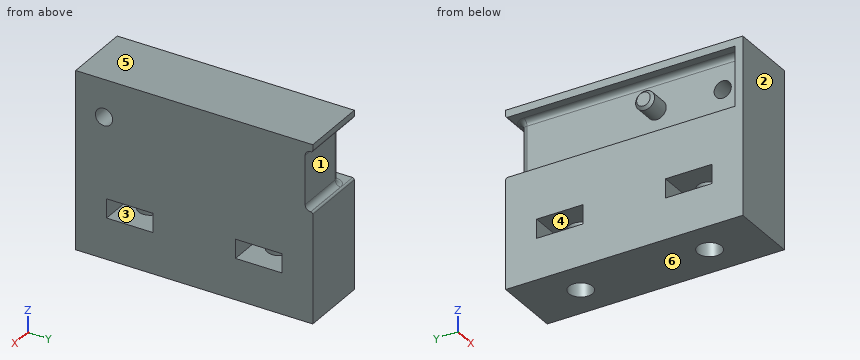
from build123d import *

# Parameters (mm, degrees)
F0_W      = 41
F0_H      = 11
F0_R      = 1.5875
F0_R_2    = 1.75
F1_DEPTH  = 10
F2_DEPTH  = 12.5
F3_R      = 1
F4_DEPTH  = 14
F5_SIZE   = 0.5
F6_DEPTH  = 19
F7_R      = 2.2
F8_DEPTH  = 20
F9_W      = 8.55
F9_H      = 3.5222247243
F10_DEPTH = 22.3


with BuildPart() as f1:
    # F0 (on Right) → F1 (new body)
    with BuildSketch(Plane.YZ):
        Rectangle(F0_W, F0_H)
        with Locations((-16.6625, 0)):
            Circle(F0_R, mode=Mode.SUBTRACT)
        with Locations((-4.475, 0)):
            Circle(F0_R_2, mode=Mode.SUBTRACT)
    extrude(amount=-F1_DEPTH)

    # F0 (on Right) → F2 (join)
    with BuildSketch(Plane.YZ):
        with BuildLine():
            Line((-20.5, 5.5), (20.5, 5.5))
            Line((20.5, 5.5), (21.5708505204, 5.5))
            ThreePointArc((21.5708505204, 5.5), (21.8035943853, 5.5964056654), (21.9000000507, 5.8291495303))
            Line((21.9000000507, 5.8291495303), (21.9000000507, 6.9000000507))
            Line((21.9000000507, 6.9000000507), (-21.9000000507, 6.9000000507))
            Line((-21.9000000507, 6.9000000507), (-21.9000000507, -6.9000000507))
            Line((-21.9000000507, -6.9000000507), (21.9000000507, -6.9000000507))
            Line((21.9000000507, -6.9000000507), (21.9000000507, -5.8291495303))
            ThreePointArc((21.9000000507, -5.8291495303), (21.8035943853, -5.5964056654), (21.5708505204, -5.5))
            Line((21.5708505204, -5.5), (20.5, -5.5))
            Line((20.5, -5.5), (-20.5, -5.5))
            Line((-20.5, -5.5), (-20.5, 5.5))
        make_face()
    extrude(amount=-F2_DEPTH)

    # F3
    f3_edges = [f1.edges().sort_by_distance(p)[0] for p in [
        (-10, 0, 5.5),
        (-10, -20.5, 0),
        (-10, 0, -5.5),
        (-10, 20.5, 0),
        (-5, 20.5, -5.5),
        (-5, 20.5, 5.5),
    ]]
    fillet(f3_edges, radius=F3_R)

    # F0 (on Right) → F4 (join)
    with BuildSketch(Plane.YZ):
        with Locations((-4.475, 0)):
            Circle(F0_R_2)
    extrude(amount=-F4_DEPTH)

    # F5
    f5_edges = [f1.edges().sort_by_distance(p)[0] for p in [
        (-14, -6.225, 0),
    ]]
    chamfer(f5_edges, length=F5_SIZE)

    # F6 (add): a face of the model
    f6_faces = [f1.faces().sort_by_distance(p)[0] for p in [
        (-6.25, 0, -6.9000000507),
    ]]
    extrude(f6_faces, amount=F6_DEPTH)

    # F7 (on face) → F8 (cut)
    with BuildSketch(Plane(origin=(0, 0, -25.9000000507), x_dir=(1, 0, 0), z_dir=(0, 0, -1))):
        with Locations((-6.1999997124, 11.8999998271)):
            Circle(F7_R)
        with Locations((-6.1999997124, -11.9000002742)):
            Circle(F7_R)
    extrude(amount=-F8_DEPTH, mode=Mode.SUBTRACT)

    # F9 (on face) → F10 (cut)
    with BuildSketch(Plane(origin=(-12.5, 0, 0), x_dir=(0, -1, 0), z_dir=(-1, 0, 0))):
        with Locations((-11.9000004627, -16.5611151606)):
            Rectangle(F9_W, F9_H)
        with Locations((11.9000000857, -16.5611151606)):
            Rectangle(F9_W, F9_H)
    extrude(amount=-F10_DEPTH, mode=Mode.SUBTRACT)


solid = f1.part
CAD build for the part. Positions are in the model's coordinates, mm. Face numbers are marked on the shaded views. A direction names the side the tool comes from. Round coordinates to 2 decimals unless told otherwise and drop trailing zeros. Write each loop counter-clockwise with the first axis right and the second up, starting at its lowest first coordinate (ties: lowest second). Pieces come first, ordered by that corner, then holes.
(1) 3-axis set-ups, long thin cutter, end or side, ignore diameter. For the marked faces 1, 2 and 3: which of +Z, -Z, +X, -X, +Y, -Y reach the whole face in a straight line?
(2) Slice it at A-A, the plane x = -11.5. Write the cut outline in (y, z) (3 decimals), and give its area (3 significant figures).
(3) Slice it at D-D, the plane z = -4. Write the cut outline in (x, y).
(4) Slice it at B-B, the plane z = 0. Write the cut outline in (x, y) (3 decimals), and give its area (4 significant figures).
(5) Slice it at C-C, the plane y = 11.9. Write the cut outline in (x, z), and give its area (3 significant figures).
(6) Probe line 1 along Y through (x, z) = (-7.75, -16) (3 decimals); line 2 along Y through (x, z) = (-6.2, -12.5); line 3 along Z through (x, y) = (-11.25, 13). List the from-to ranges inside material, lowest first.
(7) Mould opens along Z. For the marked faces 4, 5 and 6 say: pulls with the +Z half, pulls with the -Z half, needs draft (parallel to the pull), parting line crosses it, or undercut.
(8) Drop a flat-ended pin along its axis: P1, Ø3.5, axis at x = -6.2, y = 11.9, coming from the -Z side. Give the stop position or say it passes through.
From the geometry:
1. face 1: +X, -X, +Y
1. face 2: +Z, -Z, +X, -X, -Y
1. face 3: +X, -X
2. outline: (-21.9, -25.9) - (21.9, -25.9) - (21.9, -5.829) arc R0.329 ccw to (21.571, -5.5) - (-20.5, -5.5) - (-20.5, 5.5) - (21.571, 5.5) arc R0.329 ccw to (21.9, 5.829) - (21.9, 6.9) - (-21.9, 6.9) - close; circle Ø3.5 at (-4.475, 0); hole (-16.175, -18.322) - (-7.625, -18.322) - (-7.625, -14.8) - (-16.175, -14.8) - close; hole (7.625, -18.322) - (16.175, -18.322) - (16.175, -14.8) - (7.625, -14.8) - close
2. area: 920 mm2
3. outline: (-12.5, -21.9) - (0, -21.9) - (0, 20.5) - (-9, 20.5) arc R1 ccw to (-10, 19.5) - (-10, -19.5) arc R1 cw to (-11, -20.5) - (-12.5, -20.5) - close
4. outline: (-14, -5.725) - (-13.5, -6.225) - (-10, -6.225) - (-10, -15.075) - (0, -15.075) - (0, 20.5) - (-9, 20.5) arc R1 ccw to (-10, 19.5) - (-10, -2.725) - (-13.5, -2.725) - (-14, -3.225) - close; (-12.5, -21.9) - (0, -21.9) - (0, -18.25) - (-10, -18.25) - (-10, -19.5) arc R1 cw to (-11, -20.5) - (-12.5, -20.5) - close
4. area: 409.5 mm2
5. outline: (-12.5, -25.9) - (-8.4, -25.9) - (-8.4, -18.32) - (-12.5, -18.32) - close; (-12.5, -14.8) - (-8.4, -14.8) - (-8.4, -5.9) - (-4, -5.9) - (-4, -14.8) - (0, -14.8) - (0, 6.9) - (-12.5, 6.9) - (-12.5, 5.5) - (-11, 5.5) arc R1 cw to (-10, 4.5) - (-10, -4.5) arc R1 cw to (-11, -5.5) - (-12.5, -5.5) - close; (-4, -25.9) - (0, -25.9) - (0, -18.32) - (-4, -18.32) - close
5. area: 266 mm2
6. line 1: y = -21.9 to -16.175, -7.625 to 7.625, 16.175 to 21.9
6. line 2: y = -21.9 to -14.1, -9.7 to 9.7, 14.1 to 21.9
6. line 3: z = -25.9 to -18.32, -14.8 to -5.5, 5.5 to 6.9
7. face 4: undercut
7. face 5: pulls with the +Z half
7. face 6: pulls with the -Z half
8. P1: stops at z = -5.9
